from build123d import *

# Parameters (mm, degrees)
SKETCH_1_R           = 3
EXTRUDE_1_DEPTH      = 4
EXTRUDE_1_2_DEPTH    = 4
SKETCH_2_W           = 10
SKETCH_2_H           = 39.607695154
EXTRUDE_2_DEPTH      = 8
FILLET_1_R           = 3
FILLET_2_R           = 1
CUT_EXTRUDE_1_DEPTH  = 8
SKETCH_8_R           = 3
EXTRUDE_4_DEPTH      = 5
HOLE_WIZARD_M3_1_D   = 3.4
EXTRUDE_5_DEPTH      = 8
HOLE_WIZARD_M3_1_2_D = 2.5
SKETCH_10_R          = 3
CUT_EXTRUDE_2_DEPTH  = 6
CUT_EXTRUDE_3_DEPTH  = 256.457880766
SKETCH_14_R          = 7.5
EXTRUDE_6_DEPTH      = 8
FILLET_3_R           = 2
SKETCH_15_R          = 4
CUT_EXTRUDE_4_DEPTH  = 256.457880878
CUT_EXTRUDE_6_DEPTH  = 256.393399125
CUT_EXTRUDE_9_DEPTH  = 256.393399125
SKETCH_23_R          = 2
CUT_EXTRUDE_10_DEPTH = 256.393399125
SKETCH_24_R          = 3
SKETCH_24_R_2        = 1.5
EXTRUDE_7_DEPTH      = 2
FILLET_4_R           = 20
FILLET_5_R           = 1


with BuildPart() as part:
    # Sketch 1 → Extrude 1 (new, symmetric)
    with BuildSketch(Plane.XY):
        Polygon((0, -16.917096231), (7, -20.958548116), (7, -29.041451884), (0, -33.082903769), (-7, -29.041451884), (-7, -20.958548116), align=None)
        with Locations(Location((0, -25, 0), (0, 0, 180))):
            Circle(SKETCH_1_R, mode=Mode.SUBTRACT)
    extrude(amount=EXTRUDE_1_DEPTH, both=True)



with BuildPart() as body_2:
    # Sketch 1 → Extrude 1 2 (new, symmetric)
    with BuildSketch(Plane.XY):
        Polygon((7, 20.958548116), (7, 29.041451884), (0, 33.082903769), (-7, 29.041451884), (-7, 20.958548116), (0, 16.917096231), align=None)
        with Locations((0, 25)):
            Circle(SKETCH_1_R, mode=Mode.SUBTRACT)
    extrude(amount=EXTRUDE_1_2_DEPTH, both=True)


with BuildPart() as part_1:
    add(part.part)

    add(body_2.part)  # Extrude 2 merges body 2
    # Sketch 2 → Extrude 2 (add)
    with BuildSketch(Plane.XY.offset(4)):
        Rectangle(SKETCH_2_W, SKETCH_2_H)
    extrude(amount=-EXTRUDE_2_DEPTH)

    # Fillet 1
    fillet_1_edges = [part_1.edges().sort_by_distance(p)[0] for p in [
        (-5, -19.803847577, 0),
        (-5, 19.803847577, 0),
        (5, 19.803847577, 0),
        (5, -19.803847577, 0),
    ]]
    fillet(fillet_1_edges, radius=FILLET_1_R)

    # Fillet 2
    fillet_2_edges = [part_1.edges().sort_by_distance(p)[0] for p in [
        (-7, 20.958548116, 0),
        (-7, 29.041451884, 0),
        (0, 33.082903769, 0),
        (7, 29.041451884, 0),
        (7, 20.958548116, 0),
        (7, -29.041451884, 0),
        (0, -33.082903769, 0),
        (-7, -29.041451884, 0),
        (-7, -20.958548116, 0),
        (7, -20.958548116, 0),
    ]]
    fillet(fillet_2_edges, radius=FILLET_2_R - 0.0001)  # a hair under: the kernel refuses the full size

    # Sketch 3 → Cut-Extrude 1 (cut)
    with BuildSketch(Plane(origin=(0, 0, -4), x_dir=(-1, 0, 0), z_dir=(0, 0, -1))):
        with BuildLine():
            Line((-2, -15), (-2, 15))
            ThreePointArc((-2, 15), (0, 17), (2, 15))
            Line((2, 15), (2, -15))
            ThreePointArc((2, -15), (0, -17), (-2, -15))
        make_face()
    extrude(amount=-CUT_EXTRUDE_1_DEPTH, mode=Mode.SUBTRACT)

    # Sketch 8 → Extrude 4 (add)
    with BuildSketch(Plane(origin=(0, 0, -4), x_dir=(-1, 0, 0), z_dir=(0, 0, -1))):
        with Locations((0, -25)):
            Circle(SKETCH_8_R)
        with Locations((0, 25)):
            Circle(SKETCH_8_R)
    extrude(amount=-EXTRUDE_4_DEPTH)

    # Hole Wizard M3 _1 (through all)
    with Locations(Plane(origin=(0, 0, 4), x_dir=(-1, 0, 0), z_dir=(0, 0, 1))):
        with Locations((0, -25), (0, 25)):
            Hole(HOLE_WIZARD_M3_1_D / 2)

    # Sketch 9 → Extrude 5 (add)
    with BuildSketch(Plane.XY.offset(4)):
        with BuildLine():
            ThreePointArc((-24.60545694, 248.929725875), (-17.515120176, 139.163052252), (-5.674401923, 29.806786291))
            Line((-5.674401923, 29.806786291), (-0.5, 32.794228634))
            ThreePointArc((-0.5, 32.794228634), (0, 32.92820323), (0.5, 32.794228634))
            Line((0.5, 32.794228634), (4.77107276, 30.328323626))
            ThreePointArc((4.77107276, 30.328323626), (-2.557928959, 140.275299406), (-14.653344063, 249.80042293))
            ThreePointArc((-14.653344063, 249.80042293), (-20.045820832, 254.124780561), (-24.60545694, 248.929725875))
        make_face()
    extrude(amount=-EXTRUDE_5_DEPTH)

    # Hole Wizard M3 _1 2 (through all)
    with Locations(Plane.XY.offset(4)):
        with Locations((-19.610042118, 249.143807071)):
            Hole(HOLE_WIZARD_M3_1_2_D / 2)

    # Sketch 10 → Cut-Extrude 2 (cut)
    with BuildSketch(Plane.XY.offset(4)):
        with Locations((-19.610042118, 249.143807071)):
            Circle(SKETCH_10_R)
    extrude(amount=-CUT_EXTRUDE_2_DEPTH, mode=Mode.SUBTRACT)

    # Sketch 13 → Cut-Extrude 3 (cut, through all)
    with BuildSketch(Plane(origin=(0, 0, -4), x_dir=(-1, 0, 0), z_dir=(0, 0, -1))):
        with BuildLine():
            ThreePointArc((21.071643562, 237.188362315), (18.792354769, 239.797597896), (16.09460449, 237.623796811))
            ThreePointArc((16.09460449, 237.623796811), (5.322144918, 137.464104378), (-1.461601444, 36.955444756))
            ThreePointArc((-1.461601444, 36.955444756), (0.81768735, 34.346209174), (3.515437629, 36.520010259))
            ThreePointArc((3.515437629, 36.520010259), (14.287897201, 136.679702693), (21.071643562, 237.188362315))
        make_face()
    extrude(amount=-CUT_EXTRUDE_3_DEPTH, mode=Mode.SUBTRACT)

    # Sketch 14 → Extrude 6 (add)
    with BuildSketch(Plane(origin=(0, 0, -4), x_dir=(-1, 0, 0), z_dir=(0, 0, -1))):
        with Locations((9.805021059, 137.071903535)):
            Circle(SKETCH_14_R)
    extrude(amount=-EXTRUDE_6_DEPTH)

    # Fillet 3
    fillet_3_edges = [part_1.edges().sort_by_distance(p)[0] for p in [
        (-13.757410706, 130.697845481, 0),
        (-14.804208592, 142.662800065, 0),
        (-4.805833526, 131.481007005, 0),
        (-5.852631412, 143.445961589, 0),
    ]]
    fillet(fillet_3_edges, radius=FILLET_3_R)

    # Sketch 15 → Cut-Extrude 4 (cut, through all)
    with BuildSketch(Plane.XY.offset(4)):
        with Locations((-9.805021059, 137.071903535)):
            Circle(SKETCH_15_R)
    extrude(amount=-CUT_EXTRUDE_4_DEPTH, mode=Mode.SUBTRACT)

    # Sketch 16 → Cut-Extrude 6 (cut, through all)
    with BuildSketch(Plane(origin=(2.170602221, 0.189903087, 0), x_dir=(0.08715574274765833, -0.9961946980917455, 0), z_dir=(0.9961946980917455, 0.08715574274765833, 0))):
        with BuildLine():
            Line((-254.904867452, 2), (-34.904867452, 2))
            ThreePointArc((-34.904867452, 2), (-32.904867452, 0), (-34.904867452, -2))
            Line((-34.904867452, -2), (-254.904867452, -2))
            ThreePointArc((-254.904867452, -2), (-256.904867452, 0), (-254.904867452, 2))
        make_face()
    extrude(amount=CUT_EXTRUDE_6_DEPTH, mode=Mode.SUBTRACT)

    # Sketch 22 → Cut-Extrude 9 (cut, through all)
    with BuildSketch(Plane(origin=(2.170602221, 0.189903087, 0), x_dir=(0, 0, -1), z_dir=(0.9961946980917457, 0.08715574274765832, 0))):
        with BuildLine():
            Line((2, 254.904867452), (2, 219.904867452))
            ThreePointArc((2, 219.904867452), (0, 217.904867452), (-2, 219.904867452))
            Line((-2, 219.904867452), (-2, 254.904867452))
            ThreePointArc((-2, 254.904867452), (0, 256.904867452), (2, 254.904867452))
        make_face()
    extrude(amount=-CUT_EXTRUDE_9_DEPTH, mode=Mode.SUBTRACT)

    # Sketch 23 → Cut-Extrude 10 (cut, through all)
    with BuildSketch(Plane(origin=(2.170602221, 0.189903087, 0), x_dir=(0, 0, -1), z_dir=(0.9961946980917457, 0.08715574274765835, 0))):
        with Locations(Location((0, 137.404867452, 0), (0, 0, 90))):
            Circle(SKETCH_23_R)
    extrude(amount=-CUT_EXTRUDE_10_DEPTH, mode=Mode.SUBTRACT)

    # Sketch 24 → Extrude 7 (add)
    # profile 1 of 3: a face of its own
    with BuildSketch(Plane.XY.offset(4)):
        with Locations((-20.265065389, 136.156768236)):
            Circle(SKETCH_24_R)
        with Locations((-20.265065389, 136.156768236)):
            Circle(SKETCH_24_R_2, mode=Mode.SUBTRACT)
    # profile 2 of 3: a face of its own
    with BuildSketch(Plane.XY.offset(4)):
        with BuildLine():
            ThreePointArc((-17.265065389, 136.156768236), (-19.362947991, 133.295617384), (-22.722521522, 134.436038927))
            Line((-22.722521522, 134.436038927), (-16.272118562, 125.223908797))
            ThreePointArc((-16.272118562, 125.223908797), (-16.780497765, 130.820515846), (-17.276481258, 136.418235046))
            ThreePointArc((-17.276481258, 136.418235046), (-17.267920715, 136.287626188), (-17.265065389, 136.156768236))
        make_face()
    # profile 3 of 3: a face of its own
    with BuildSketch(Plane.XY.offset(4)):
        with BuildLine():
            Line((-17.53520033, 139.395600482), (-20.265065389, 139.156768236))
            ThreePointArc((-20.265065389, 139.156768236), (-18.238294611, 138.368600105), (-17.276481258, 136.418235046))
            ThreePointArc((-17.276481258, 136.418235046), (-17.406279124, 137.906879675), (-17.53520033, 139.395600482))
        make_face()
    extrude_7 = extrude(amount=-EXTRUDE_7_DEPTH)

    # Mirror 1: Extrude 7 across plane
    add(extrude_7.mirror(Plane.XY))

    # Fillet 4
    fillet_4_edges = [part_1.edges().sort_by_distance(p)[0] for p in [
        (-16.272118562, 125.223908797, 3),
        (-16.272118562, 125.223908797, -3),
    ]]
    fillet(fillet_4_edges, radius=FILLET_4_R)

    # Fillet 5
    fillet_5_edges = [part_1.edges().sort_by_distance(p)[0] for p in [
        (-17.53520033, 139.395600482, 3),
        (-17.53520033, 139.395600482, -3),
    ]]
    fillet(fillet_5_edges, radius=FILLET_5_R)


solid = part_1.part
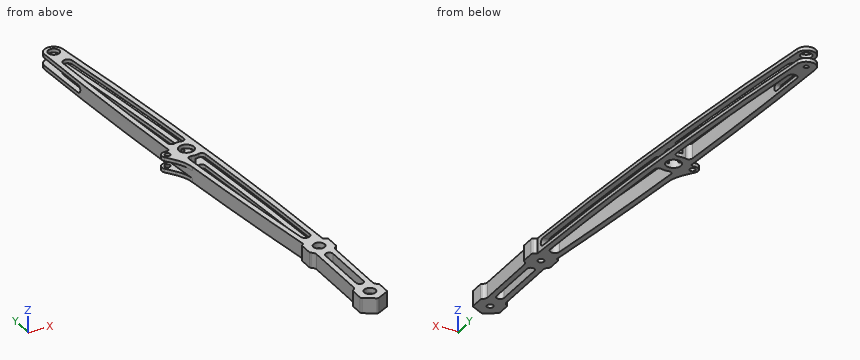
Model file for the job. Use its own axes, mm. Give positions to 0.01 mm unless a question says otherwise; leave off trailing zeros. Order: outer loops, then holes, each group sorted by start corner. A loop starts at its lowest first (then second) coordinate and runs counter-clockwise, first axis right, second up. Notation, with made-up numbers: (30.5, -26) -> (50.5, -26) arc R20 cw to (50.5, 6) -> close; hole circle Ø6 at (-31, 40). An arc over 180 degrees is marked (long way). Use CSV: the item, a comma, the result in double quotes.
1. Drill centre lines: line 1 along Z through (x, y) = (2, 56.5); line 2 along X through (y, z) = (-25, -1.45); line 3 along X through (y, z) = (-1, 2). Where is each one in solid material? Low to high. Write a range as from..to.
Outcome:
line 1,"-4..-2, 2..4"
line 2,"-7..-1.7, 1.7..7"
line 3,"-5..-2, 2..5"
2. Drop flat-ended pins along their axis: pin 1 (1.8 mm diameter, centred on x = -20.27, y = 136.16, fed in from -Z); pin 2 (5 mm diameter, centred on x = 0, y = -25, fed in from +Z); pin 3 (4 mm diameter, centred on y = -5.5, z = -1.5, fed in from +X); pin 4 (2.5 mm diameter, centred on y = -8, z = -1.5, fed in from -X). Give the stop position or say it passes through.
Outcome:
pin 1,"through"
pin 2,"z = 1"
pin 3,"x = 5"
pin 4,"x = -5"
3. Band-saw the part on A-A, the plane y = 162.5. Give the cut face in (x, z).
Outcome:
outline,"(-19.42, -4) -> (-16.41, -4) -> (-16.41, 4) -> (-19.42, 4) -> close; (-7.64, -4) -> (-4.62, -4) -> (-4.62, -2) -> (-7.64, -2) -> close; (-7.64, 2) -> (-4.62, 2) -> (-4.62, 4) -> (-7.64, 4) -> close"
4. Band-saw the part on B-B, the plane y = 203. Give the cut face in (x, z).
Outcome:
outline,"(-22.22, -4) -> (-19.21, -4) -> (-19.21, 4) -> (-22.22, 4) -> close; (-11.91, -4) -> (-8.9, -4) -> (-8.9, -2) -> (-11.91, -2) -> close; (-11.91, 2) -> (-8.9, 2) -> (-8.9, 4) -> (-11.91, 4) -> close"
